Input: part model. Units: mm. Frame: model coordinates. Round coordinates to 2 decimals unless told otherwise and drop trailing zeros. Write each loop counter-clockwise with the first axis right and the second up, starting at its lowest first coordinate (ties: lowest second). Pieces come first, ordered by that corner, then holes. Notation, with made-up numbers: (-19.75, 4.5) - (3.25, 4.5) arc R27 cw to (3.25, 39.5) - close; hole circle Ø3 at (8, -34.75). An arc over 180 degrees is marked (long way). One line per item, written item: value. Start each with the question number.
```python
from build123d import *

# Parameters (mm, degrees)
CROQUIS1_W              = 20
CROQUIS1_H              = 6
SALIENTE_EXTRUIR1_DEPTH = 30
CROQUIS2_R              = 1.5
CORTAR_EXTRUIR1_DEPTH   = 5
CROQUIS3_R              = 1.5
CORTAR_EXTRUIR3_DEPTH   = 5
CROQUIS4_R              = 0.5
CORTAR_EXTRUIR4_DEPTH   = 10


with BuildPart() as part:
    # Croquis1 → Saliente-Extruir1 (new body)
    with BuildSketch(Plane.XY):
        with Locations((10, 3)):
            Rectangle(CROQUIS1_W, CROQUIS1_H)
    extrude(amount=SALIENTE_EXTRUIR1_DEPTH)

    # Croquis2 → Cortar-Extruir1 (cut)
    with BuildSketch(Plane.XY.offset(30)):
        with Locations((3, 3)):
            Circle(CROQUIS2_R)
        with Locations((17, 3)):
            Circle(CROQUIS2_R)
    extrude(amount=-CORTAR_EXTRUIR1_DEPTH, mode=Mode.SUBTRACT)

    # Croquis3 → Cortar-Extruir3 (cut)
    with BuildSketch(Plane(origin=(0, 0, 0), x_dir=(-1, 0, 0), z_dir=(0, 0, -1))):
        with Locations((-17, 3)):
            Circle(CROQUIS3_R)
        with Locations((-3, 3)):
            Circle(CROQUIS3_R)
    extrude(amount=-CORTAR_EXTRUIR3_DEPTH, mode=Mode.SUBTRACT)

    # Croquis4 → Cortar-Extruir4 (cut)
    with BuildSketch(Plane(origin=(0, 6, 0), x_dir=(1, 0, 0), z_dir=(0, 1, 0))):
        with Locations((15, -11)):
            Circle(CROQUIS4_R)
    extrude(amount=-CORTAR_EXTRUIR4_DEPTH, mode=Mode.SUBTRACT)


solid = part.part
```
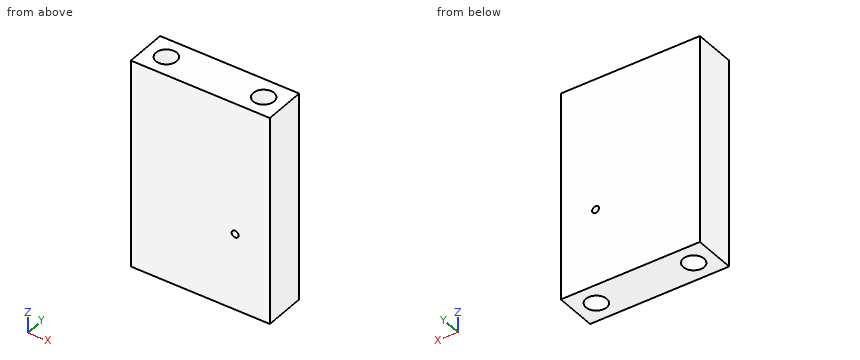
Q1. Cut plane C-C, the plane y = 3. Output: boundary loops of the cut face in (x, z).
Q2. Material intervals for probe 1 along Z at (x, y) = (15, 3.95); probe 2 along X at (y, z) = (1.75, 11); probe 3 along Y at (x, z) = (3, 2.5), sorted ascending. Write a range as from..to.
Q3. Contact query for flat-ended pins moving along their axis: pin 1 Ø0.9 at (x, y) = (3, 3.5) entering from +Z; pin 2 Ø1.8 at (x, y) = (3, 3) entering from -Z. Output: stop coordinate, or through.
Q4. Cut plane B-B, the plane x = 15. Output: boundary loops of the cut face in (y, z).
Q5. Cut plane D-D, the plane x = 17. Output: boundary loops of the cut face in (y, z).
Q6. Cut plane A-A, the plane z = 11. Output: boundary loops of the cut face in (x, y).
A:
1. outline: (0, 0) - (1.5, 0) - (1.5, 5) - (4.5, 5) - (4.5, 0) - (15.5, 0) - (15.5, 5) - (18.5, 5) - (18.5, 0) - (20, 0) - (20, 30) - (18.5, 30) - (18.5, 25) - (15.5, 25) - (15.5, 30) - (4.5, 30) - (4.5, 25) - (1.5, 25) - (1.5, 30) - (0, 30) - close; hole circle Ø1 at (15, 11)
2. probe 1: z = 0..10.5, 11.5..30
2. probe 2: x = 0..14.5, 15.5..20
2. probe 3: y = 0..1.5, 4.5..6
3. pin 1: stops at z = 25
3. pin 2: stops at z = 5
4. outline: (0, 0) - (6, 0) - (6, 10.5) - (0, 10.5) - close; (0, 11.5) - (6, 11.5) - (6, 30) - (0, 30) - close
5. outline: (0, 0) - (1.5, 0) - (1.5, 5) - (4.5, 5) - (4.5, 0) - (6, 0) - (6, 30) - (4.5, 30) - (4.5, 25) - (1.5, 25) - (1.5, 30) - (0, 30) - close
6. outline: (0, 0) - (14.5, 0) - (14.5, 6) - (0, 6) - close; (15.5, 0) - (20, 0) - (20, 6) - (15.5, 6) - close
